Here's how the part is built. I have some questions about the finished solid (model axes, mm). Face numbers are marked on the shaded views. A direction names the side the tool comes from. Round coordinates to 2 decimals unless told otherwise and drop trailing zeros. Write each loop counter-clockwise with the first axis right and the second up, starting at its lowest first coordinate (ties: lowest second). Pieces come first, ordered by that corner, then holes. Notation, with made-up numbers: M 14.25,-37 L 67.25,-37 A17 cw 67.25,-7 Z; hole C 4,-9 d11. An arc over 180 degrees is marked long. Use a Markdown table: item, result. Add a question column.
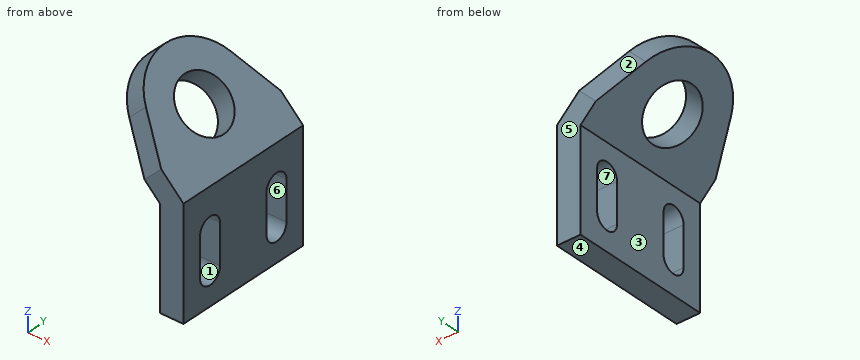
```python
from build123d import *

# Parameters (mm, degrees)
F1_DEPTH = 72
F2_R     = 14
F3_DEPTH = 25
F6_DEPTH = 25
F8_DEPTH = 25


with BuildPart() as f1:
    # F0 (on Front) → F1 (new body)
    with BuildSketch(Plane.XZ):
        Polygon((26.0169860537, -41.8088145156), (26.0169860537, 14.1911854844), (-13.5809936927, 53.7891652309), (-22.066275067, 45.3038838566), (14.0169860537, 9.2206227359), (14.0169860537, -41.8088145156), align=None)
    extrude(amount=F1_DEPTH)

    # F2 (on face) → F3 (cut)
    with BuildSketch(Plane(origin=(20.1040857691, 0, 20.1040857691), x_dir=(0.7071067812, 0, -0.7071067812), z_dir=(0.7071067812, 0, 0.7071067812))):
        with Locations((-19.6378962245, -36)):
            Circle(F2_R)
    extrude(amount=-F3_DEPTH, mode=Mode.SUBTRACT)

    # F5 (on face) + F4 (on face) → F6 (cut)
    with BuildSketch(Plane(origin=(20.1040857691, 0, 20.1040857691), x_dir=(0.7071067812, 0, -0.7071067812), z_dir=(0.7071067812, 0, 0.7071067812))):
        Polygon((-47.6378962245, -17.821869662), (-31.0333128979, -10.4237516661), (-7.6378962245, 0), (-47.6378962245, 0), align=None)
        Polygon((-47.6378962245, -72), (-7.6378962245, -72), (-31.0333098725, -61.5762496819), (-47.6378962245, -54.178130338), align=None)
        with BuildLine():
            Line((-47.6378962245, -54.178130338), (-31.0333098725, -61.5762496819))
            ThreePointArc((-31.0333098725, -61.5762496819), (-43.1226953736, -51.2467770013), (-47.6378962245, -36))
            Line((-47.6378962245, -36), (-47.6378962245, -54.178130338))
        make_face()
    with BuildSketch(Plane(origin=(20.1040857691, 0, 20.1040857691), x_dir=(0.7071067812, 0, -0.7071067812), z_dir=(0.7071067812, 0, 0.7071067812))):
        with BuildLine():
            Line((-31.0333129323, -10.4237516814), (-88.4374995943, -36))
            Line((-88.4374995943, -36), (-31.0333096209, -61.576249794))
            ThreePointArc((-31.0333096209, -61.576249794), (-43.1226952986, -51.2467771168), (-47.6378962245, -36))
            ThreePointArc((-47.6378962245, -36), (-43.1226962856, -20.7532244035), (-31.0333129323, -10.4237516814))
        make_face()
    extrude(amount=-F6_DEPTH, mode=Mode.SUBTRACT)

    # F7 (on face) → F8 (cut)
    with BuildSketch(Plane.YZ.offset(26.0169860537)):
        with BuildLine():
            ThreePointArc((-62, -25.8088145156), (-56, -31.8088145156), (-50, -25.8088145156))
            ThreePointArc((-50, -25.8088145156), (-56, -19.8088145156), (-62, -25.8088145156))
        make_face()
        with BuildLine():
            ThreePointArc((-62, -25.8088145156), (-56, -19.8088145156), (-50, -25.8088145156))
            Line((-50, -25.8088145156), (-50, -5.8088145156))
            ThreePointArc((-50, -5.8088145156), (-56, -11.8088145156), (-62, -5.8088145156))
            Line((-62, -5.8088145156), (-62, -25.8088145156))
        make_face()
        with BuildLine():
            ThreePointArc((-62, -5.8088145156), (-56, -11.8088145156), (-50, -5.8088145156))
            ThreePointArc((-50, -5.8088145156), (-56, 0.1911854844), (-62, -5.8088145156))
        make_face()
        with BuildLine():
            Line((-22, -25.8088145156), (-10, -25.8088145156))
            ThreePointArc((-10, -25.8088145156), (-16, -19.8088145156), (-22, -25.8088145156))
        make_face()
        with BuildLine():
            ThreePointArc((-22, -25.8088145156), (-16, -31.8088145156), (-10, -25.8088145156))
            Line((-10, -25.8088145156), (-22, -25.8088145156))
        make_face()
        with BuildLine():
            ThreePointArc((-22, -25.8088145156), (-16, -19.8088145156), (-10, -25.8088145156))
            Line((-10, -25.8088145156), (-10, -5.8088145156))
            ThreePointArc((-10, -5.8088145156), (-16, -11.8088145156), (-22, -5.8088145156))
            Line((-22, -5.8088145156), (-22, -25.8088145156))
        make_face()
        with BuildLine():
            ThreePointArc((-22, -5.8088145156), (-16, -11.8088145156), (-10, -5.8088145156))
            ThreePointArc((-10, -5.8088145156), (-16, 0.1911854844), (-22, -5.8088145156))
        make_face()
    extrude(amount=-F8_DEPTH, mode=Mode.SUBTRACT)


solid = f1.part
```
Item 1: Imagine slicing it at A-A on y = -57. List the corners of the cut face in (x, z) for me, plus the area to 3 significant figures.
Item 2: For pin 1 Ø10 at (x, y) = (4, -35.5) entering from -Z; pin 2 Ø1.5 at (y, z) = (-61.5, -2) entering from -X; pin 3 Ø4 at (x, y) = (-12.5, -59) entering from -Z, each with a flat end and sliding along its axis, tell me the tip position at first contact or that it passes through.
Item 3: If we mould it in two halves opening along Z, with no side actions, what happens to the marked faces 4, 5, 6 and 7? For each: +Z half, -Z half, draft (parallel to the pull), parting line (faces both ways), or undercut.
Item 4: On a 3-axis mill with a long thin cutter (end or side, diameter ignored), from which of +Z, -Z, +X, -X, +Y, -Y can I reach the whole of each face in a straight line? I mean the marked faces 1, 2 and 3. Say none if no direction works.
Item 5: Imagine slicing it at B-B on z = 5. List the corners of the cut face in (x, y) for me.
Item 6: I need wall thicknesses on probe 1 along Y at (x, z) = (19, -0.5); probe 2 along Y at (x, z) = (-2.5, 38); probe 3 along X at (y, z) = (-40, -1). Which ranges of each line are inside material? Lowest first, please. Write a range as from..to.
Item 7: Imagine slicing it at C-C on y = -16. List the corners of the cut face in (x, z) for me, plus the area to 3 significant figures.
The answers:
| question | item | result |
|---|---|---|
| 1 | outline | M -15.36,38.6 L 14.02,9.22 L 14.02,0.11 L 26.02,0.11 L 26.02,14.19 L -6.88,47.09 Z; M 14.02,-41.81 L 26.02,-41.81 L 26.02,-31.72 L 14.02,-31.72 Z |
| 1 | area | 789 mm² |
| 2 | pin 1 | z = 14.24 |
| 2 | pin 2 | x = 14.02 |
| 2 | pin 3 | z = 33.74 |
| 3 | face 4 | -Z half |
| 3 | face 5 | draft |
| 3 | face 6 | undercut |
| 3 | face 7 | undercut |
| 4 | face 1 | +X, -X |
| 4 | face 2 | +Z, -X, +Y |
| 4 | face 3 | -Z, -X, +Y, -Y |
| 5 | outline | M 14.02,-72 L 26.02,-72 L 26.02,0 L 14.02,0 Z |
| 6 | probe 1 | -72..-58.8, -53.2..-18.8, -13.2..0 |
| 6 | probe 2 | -62.64..-46.72, -25.28..-9.36 |
| 6 | probe 3 | 14.02..26.02 |
| 7 | outline | M -16.12,39.36 L 14.02,9.22 L 14.02,0.19 L 26.02,0.19 L 26.02,14.19 L -7.64,47.85 Z; M 14.02,-41.81 L 26.02,-41.81 L 26.02,-31.81 L 14.02,-31.81 Z |
| 7 | area | 800 mm² |
